```python
from build123d import *

# Parameters (mm, degrees)
F2_R    = 2.99999
F3_R    = 2.99999
F4_R    = 1.49999
F5_SIZE = 1


# Not quite as in the source:
# - a fillet or chamfer is up to 0.001 mm smaller than in the source, because OpenCascade refuses the exact size


with BuildPart() as f1:
    # F0 (on Front) → F1 (revolve)
    with BuildSketch(Plane.XZ):
        Polygon((30.25, 0), (33.25, 0), (33.25, 55), (30.25, 55), (30.25, 17), (27.25, 17), (27.25, 15), (30.25, 15), align=None)
    revolve(axis=Axis((0, 0, 28.8916025311), (0, 0, 1)))

    # F2 (radius 3 in the source; OpenCascade refuses exactly that, so slightly less here)
    f2_edges = [f1.edges().sort_by_distance(p)[0] for p in [
        (-30.25, 0, 17),
    ]]
    fillet(f2_edges, radius=F2_R)

    # F3 (radius 3 in the source; OpenCascade refuses exactly that, so slightly less here)
    f3_edges = [f1.edges().sort_by_distance(p)[0] for p in [
        (-30.25, 0, 15),
    ]]
    fillet(f3_edges, radius=F3_R)

    # F4 (radius 1.5 in the source; OpenCascade refuses exactly that, so slightly less here)
    f4_edges = [f1.edges().sort_by_distance(p)[0] for p in [
        (-30.25, 0, 55),
        (-33.25, 0, 55),
    ]]
    fillet(f4_edges, radius=F4_R)

    # F5
    f5_edges = [f1.edges().sort_by_distance(p)[0] for p in [
        (-33.25, 0, 0),
    ]]
    chamfer(f5_edges, length=F5_SIZE)


solid = f1.part
```
Work out the finished part from the listing and answer in its coordinate system (mm). A direction names the side the tool comes from. Give positions to 0.01 mm unless a question says otherwise; leave off trailing zeros. Order: outer loops, then holes, each group sorted by start corner. A loop starts at its lowest first (then second) coordinate and runs counter-clockwise, first axis right, second up. Notation, with made-up numbers: (46, -22) - (66, -22) arc R22 cw to (66, -1) - close; hole circle Ø9 at (-7, 43.25). An arc over 180 degrees is marked (long way). One line per item, written item: value. Start each with the question number.
1. Each of these flat-tipped pins is pushed along its axis until it touches: pin 1 Ø10 at (x, z) = (-5.5, 47.5) entering from -Y; pin 2 Ø5 at (x, z) = (0.5, 45.5) entering from +Y; pin 3 Ø10 at (x, z) = (14, 48) entering from -Y. Where does it stop, or does it pass through?
2. Consider line 1 (Y direction, x = 0, z = 16); line 2 (X direction, y = -1, z = 38); line 3 (Y direction, x = 0, z = 43.5). Determine where each line is inside the solid, lowest interval first.
3. For a pull along Y with two mould halves and no side action, classify faces 1 (the face through (10, 29, 0)), 2 (the face through (17.87, 28.04, 27.62)), 3 (the face through (-6.56, -29.53, 36.52)) as released by +Y, released by -Y, zero draft, split by the parting line, or undercut.
4. Section C-C, the plane z = 49 is taken. Write down the section's boundary in (x, y), then the cut area to 3 significant figures.
5. Which of the six approach directions +Z, -Z, +X, -X, +Y, -Y give full straight-line access (tool end or side, diameter ignored) to faces 4 (the face through (-21.625, -16.581, 15.986)), 5 (the face through (-6.56, -29.53, 5.92))?
Filled sheet:
1. pin 1: y = -33.25
1. pin 2: y = 33.25
1. pin 3: y = -32.01
2. line 1: -33.25 to -27.25, 27.25 to 33.25
2. line 2: -33.23 to -30.23, 30.23 to 33.23
2. line 3: -33.25 to -30.25, 30.25 to 33.25
3. face 1: zero draft
3. face 2: split by the parting line
3. face 3: undercut
4. outline: circle Ø66.5 at (0, 0); hole circle Ø60.5 at (0, 0)
4. area: 598 mm²
5. face 4: +Z, -Z
5. face 5: -Z
